Design review of the part shown in the three views and the two pictorial views. Dimensions are in mm from the part's minimum x, y and z. Coordinates: 2 decimals unless noted, no trailing zeros. Loops run counter-clockwise (first coordinate to the right, second up) from the corner with the lowest first, then second, coordinate; pieces in that order, holes last. Notation, with made-up numbers: M 2.25,77 L 50.25,77 A10 cw 50.25,90 Z; hole C 33.25,46 d1. An arc over 180 degrees is marked long. Put each result on its own line as item: value. Start each with the question number.
(1) Take a section at C-C, the plane z = 4. Give the boundary of the cut face in (x, y) (1 decimal), then the cut area to 3 significant figures.
(2) Take a section at A-A, the plane y = 40. Give the boundary of the cut face in (x, z), then the cut area to 3 significant figures.
(3) For probe 1 along Y at (x, z) = (10, 2); probe 2 along X at (y, z) = (35, 3.1); probe 3 along Y at (x, z) = (41, 2.8), list the stretches that pass through material, from the lowest coordinate up. Write a range as [from, to].
(4) Clearance check with a flat-ended pin moving along its axis: pin 1 (8 mm diameter, centred on x = 14.98, y = 35.67, fed in from +Z). State where the tip first meets the part, or that it passes through.
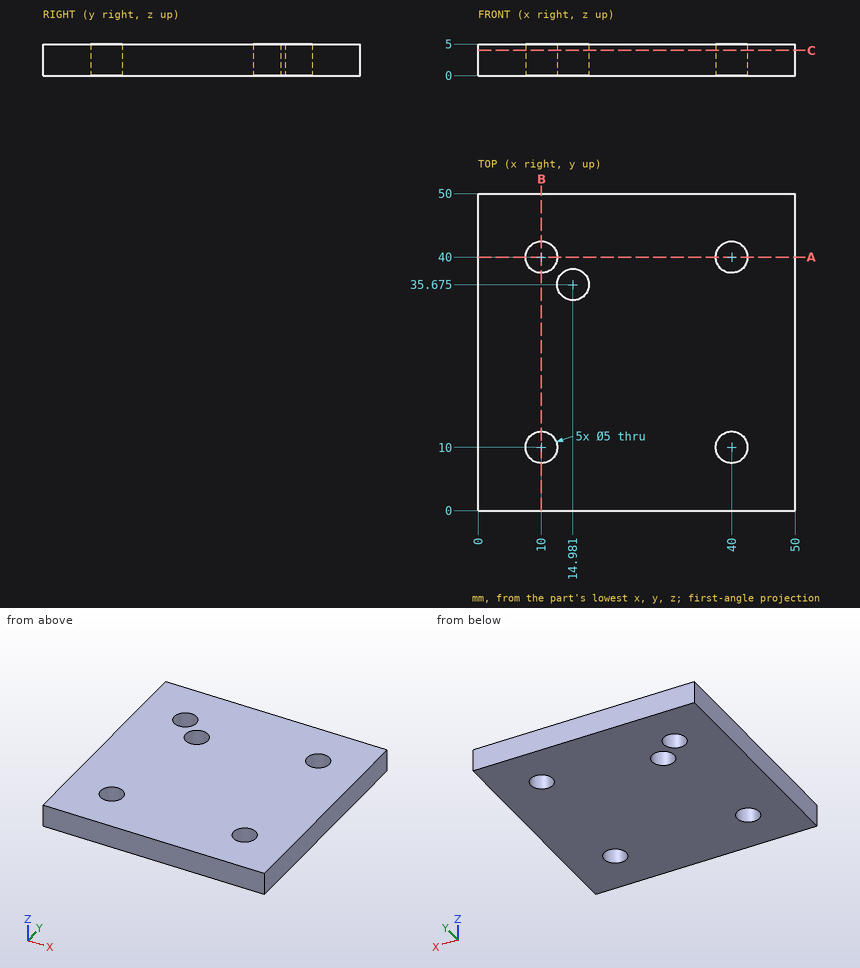
Computed values:
1. outline: M 0,0 L 50,0 L 50,50 L 0,50 Z; hole C 10,10 d5; hole C 10,40 d5; hole C 15,35.7 d5; hole C 40,10 d5; hole C 40,40 d5
1. area: 2,400 mm^2
2. outline: M 0,0 L 7.5,0 L 7.5,5 L 0,5 Z; M 12.5,0 L 37.5,0 L 37.5,5 L 12.5,5 Z; M 42.5,0 L 50,0 L 50,5 L 42.5,5 Z
2. area: 200 mm^2
3. probe 1: y = [0, 7.5], [12.5, 37.5], [42.5, 50]
3. probe 2: x = [0, 12.57], [17.39, 50]
3. probe 3: y = [0, 7.71], [12.29, 37.71], [42.29, 50]
4. pin 1: stops at z = 5
